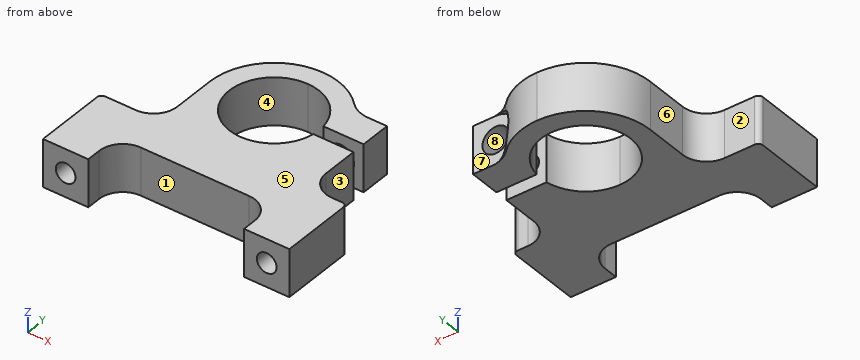
Autodesk Inventor part; units mm, degrees
ref_plane "YZ Plane" through (0, 0, 0) normal (1, 0, 0) x (0, 1, 0)
ref_plane "XZ Plane" through (0, 0, 0) normal (0, 1, 0) x (-1, 0, 0)
ref_plane "XY Plane" through (0, 0, 0) normal (0, 0, 1) x (1, 0, 0)
sketch "Sketch1" plane through (0, 0, 0) normal (0, 0, 1) x (1, 0, 0)
  line L0 (0, 0) -> (0, 14.864) construction
  arc A0 (0, 25.05) -> (0, 13.05) centre (0, 19.05) ccw
  line L1 (-10.4394, 0) -> (-10.4394, 1.905)
  line L2 (-7.2644, 5.08) -> (0, 5.08)
  line L3 (-16.51, 0) -> (-16.51, 9.525)
  line L4 (-15.875, 10.16) -> (-11.811, 10.16)
  line L5 (-8.636, 13.335) -> (-8.636, 19.05)
  arc A1 (0, 27.686) -> (-8.636, 19.05) centre (0, 19.05) ccw
  arc A2 (-7.2644, 5.08) -> (-10.4394, 1.905) centre (-7.2644, 1.905) ccw
  line L6 (-10.4394, 0) -> (-16.51, 0)
  arc A3 (-15.875, 10.16) -> (-16.51, 9.525) centre (-15.875, 9.525) ccw
  arc A4 (-11.811, 10.16) -> (-8.636, 13.335) centre (-11.811, 13.335) ccw
  arc A5 (5.9338, 19.939) -> (0, 25.05) centre (0, 19.05) ccw
  arc A6 (0, 13.05) -> (5.9338, 18.161) centre (0, 19.05) ccw
  arc A7 (6.0886, 25.1745) -> (0, 27.686) centre (0, 19.05) ccw
  line L7 (8.7747, 24.0665) -> (11.3186, 24.0665)
  line L8 (11.3186, 24.0665) -> (11.3186, 19.939)
  line L9 (11.3186, 19.939) -> (5.9338, 19.939)
  line L10 (5.9338, 18.161) -> (11.3186, 18.161)
  line L11 (11.3186, 18.161) -> (11.3186, 13.335)
  line L12 (14.4936, 10.16) -> (15.875, 10.16)
  line L13 (16.51, 9.525) -> (16.51, 0)
  line L14 (16.51, 0) -> (10.4394, 0)
  line L15 (10.4394, 0) -> (10.4394, 1.905)
  line L16 (7.2644, 5.08) -> (0, 5.08)
  arc A8 (10.4394, 1.905) -> (7.2644, 5.08) centre (7.2644, 1.905) ccw
  arc A9 (11.3186, 13.335) -> (14.4936, 10.16) centre (14.4936, 13.335) ccw
  arc A10 (16.51, 9.525) -> (15.875, 10.16) centre (15.875, 9.525) ccw
  line L17 (0, 19.05) -> (12.673, 19.05) construction
  arc A11 (6.0886, 25.1745) -> (8.7747, 24.0665) centre (8.7747, 27.8765) ccw
  point P0 (7.0296, 24.0665)
  dimension "d0" = 19.05
  dimension "d1" = 6
  dimension "d2" = 27.686
  dimension "d3" = 3.175
  dimension "d4" = 0.635
  dimension "d5" = 3.175
  dimension "d6" = 33.02
  dimension "d7" = 10.16
  dimension "d8" = 6.0706
  dimension "d9" = 5.08
  dimension "d10" = 3.175
  dimension "d11" = 0.635
  dimension "d12" = 5.3848
  dimension "d13" = 1.778
  dimension "d14" = 3.81
  dimension "d15" = 4.1275
extrude "Extrusion1" add sketch "Sketch1" along normal blind 6.35
sketch "Sketch3" plane through (8.7747, 24.0665, 0) normal (0, 1, 0) x (1, 0, 0)
  line L0 (0, 0) -> (2.5438, 0)
  line L1 (2.5438, -6.35) -> (0, -6.35)
  line L2 (2.5438, 0) -> (2.5438, -6.35)
  line L3 (2.5438, -3.175) -> (-0.5042, -3.175) construction
  line L4 (0, 0) -> (-0.5042, 0)
  line L5 (0, -6.35) -> (-0.5042, -6.35)
  arc A0 (-0.5042, 0) -> (-0.5042, -6.35) centre (-0.5042, -3.175) ccw
  point P0 (-8.7747, 0)
  dimension "d22" = 3.048
extrude "Extrusion2" cut sketch "Sketch3" along normal blind 6.35
sketch "Sketch4" plane through (11.3186, 24.0665, 6.35) normal (0, 1, 0) x (1, 0, 0)
  arc A0 (-3.048, 6.35) -> (-3.048, 0) centre (-3.048, 3.175) ccw
  point P0 (-11.3186, 6.35)
hole "Hole1" at (8.2706, 24.0665, 3.175) direction (0, -1, 0) diameter 3.556 depth 5.08
sketch "Sketch5" plane through (5.9338, 18.161, 0) normal (0, 1, 0) x (1, 0, 0)
  circle A0 centre (2.3368, -3.175) radius 1.778
  point P0 (-5.9338, 0)
hole "Hole2" at (8.2706, 18.161, 3.175) direction (0, -1, 0) diameter 2.6416 depth 6.35 tip angle 118
sketch "Sketch6" plane through (-16.51, 0, 0) normal (0, -1, 0) x (1, 0, 0)
  line L0 (33.02, 0) -> (26.9494, 0)
  line L1 (33.02, 0) -> (33.02, 6.35)
  line L2 (26.9494, 6.35) -> (33.02, 6.35)
  line L3 (26.9494, 0) -> (26.9494, 6.35)
  line L4 (0, 0) -> (6.0706, 6.35) construction
  line L5 (26.9494, 0) -> (33.02, 6.35) construction
  point P0 (16.51, 0)
  point P1 (3.0353, 3.175)
  point P2 (29.9847, 3.175)
hole "Hole3" at (-13.4747, 0, 3.175) at (13.4747, 0, 3.175) direction (0, 1, 0) diameter 2.6416 depth 8.89 tip angle 118
properties part number "535638-12mmClampingBracket"
Geometry check sheet. Reference: the model listing, model coordinates, mm. Face numbers are marked on the shaded views. A direction names the side the tool comes from. Round coordinates to 2 decimals unless told otherwise and drop trailing zeros. Order: outer loops, then holes, each group sorted by start corner. A loop starts at its lowest first (then second) coordinate and runs counter-clockwise, first axis right, second up. Notation, with made-up numbers: (18, 43.25) - (24, 43.25) arc R24 ccw to (24, 70.25) - close; hole circle Ø6 at (-29, -9). An arc over 180 degrees is marked (long way). Use a Markdown table: item, result. Add a question column.
1) Section check B-B (y = 16.75). Record the cut outline in (x, z) (3 decimals).
2) Section check C-C (y = 8). Record the cut outline in (x, z) (3 decimals).
3) Gauge pin test, flat ends, axial feed: P1, Ø3, axis at x = 6.5, z = 3, coming from the -Y side; P2, Ø2.5, axis at y = 16, z = 3.5, coming from the +X side; P3, Ø3, axis at x = 13.47, z = 3.18, coming from the +Y side. Record the tip position at first contact, or that the pin passes through.
4) Mould release check, pull along Z, two halves, no side actions. Record for the marked faces 5, 6, 7 and 8: released by +Z, released by -Z, zero draft, split by the parting line, or undercut.
5) Section check A-A (x = 2). Record the cut outline in (y, z).
6) Set-up check for the marked faces 1, 2, 3 and 4: record each of +Z, -Z, +X, -X, +Y, -Y from which the full face is reachable in a straight line by a thin tool's end or side.
7) Thickness scan on line 1 along X through (y, z) = (14.75, 3.75); line 2 along X through (y, z) = (16.75, 2.5); line 3 along X through (y, z) = (2.5, 3). Record the ranges inside material, lowest first.
Established:
| question | item | result |
|---|---|---|
| 1 | outline | (-8.636, 0) - (-5.542, 0) - (-5.542, 6.35) - (-8.636, 6.35) - close; (5.542, 0) - (11.319, 0) - (11.319, 6.35) - (5.542, 6.35) - close; hole circle Ø2.642 at (8.271, 3.175) |
| 2 | outline | (-16.51, 0) - (16.51, 0) - (16.51, 6.35) - (-16.51, 6.35) - close; hole circle Ø2.642 at (-13.475, 3.175); hole circle Ø2.642 at (13.475, 3.175) |
| 3 | P1 | y = 4.99 |
| 3 | P2 | x = 11.32 |
| 3 | P3 | y = 11.41 |
| 4 | face 5 | released by +Z |
| 4 | face 6 | zero draft |
| 4 | face 7 | undercut |
| 4 | face 8 | undercut |
| 5 | outline | (5.08, 0) - (13.39, 0) - (13.39, 6.35) - (5.08, 6.35) - close; (24.71, 0) - (27.45, 0) - (27.45, 6.35) - (24.71, 6.35) - close |
| 6 | face 1 | +Z, -Z, -Y |
| 6 | face 2 | +Z, -Z, -X, +Y |
| 6 | face 3 | +Z, -Z, +X, +Y |
| 6 | face 4 | +Z, -Z |
| 7 | line 1 | -8.64 to -4.18, 4.18 to 7.08, 9.46 to 11.32 |
| 7 | line 2 | -8.64 to -5.54, 5.54 to 7.14, 9.41 to 11.32 |
| 7 | line 3 | -16.51 to -14.78, -12.17 to -10.38, 10.38 to 12.17, 14.78 to 16.51 |
